Check sheet for the modelled part. Datum: model origin and axes. Units: mm. A direction names the side the tool comes from. Round coordinates to 2 decimals unless told otherwise and drop trailing zeros. Order: outer loops, then holes, each group sorted by start corner. A loop starts at its lowest first (then second) coordinate and runs counter-clockwise, first axis right, second up.
```python
from build123d import *

# Parameters (mm, degrees)
F2_R = 0.13


# Not quite as in the source:
# - a feature names something its author has since deleted; it is built from what else it names


with BuildPart() as f1:
    # F0 (on Top) → F1 (revolve)
    with BuildSketch(Plane.XY):
        with BuildLine():
            Line((7.3, 15.1), (7.3, 22.16))
            Line((7.3, 22.16), (1.6, 22.16))
            Line((1.6, 22.16), (1.6, 20.79))
            Line((1.6, 20.79), (2.9, 20.79))
            Line((2.9, 20.79), (2.9, 19.05))
            Line((2.9, 19.05), (3.16, 19.05))
            ThreePointArc((3.16, 19.05), (5.2813203436, 18.1713203436), (6.16, 16.05))
            Line((6.16, 16.05), (6.16, 15.1))
            Line((6.16, 15.1), (7.3, 15.1))
        make_face()
    revolve(axis=Axis((7.0380799007, 0, 0), (1, 0, 0)))

    # F2
    f2_edges = [f1.edges().sort_by_distance(p)[0] for p in [
        (7.3, -22.16, 0),
        (1.6, -22.16, 0),
        (1.6, -20.79, 0),
    ]]
    fillet(f2_edges, radius=F2_R)


solid = f1.part
```
Item 1: Sectioned sample at C-C (x = 5.55). Record the cut outline in (y, z), and give its area (3 significant figures).
Answer:
outline: circle Ø44.32 at (0, 0); hole circle Ø35.73 at (0, 0)
area: 540 mm2
Item 2: Release check for a two-part mould opening along Z. For faces 3 (the cylindrical face through (2.32, 19.83, 6.24)), 4 (the cylindrical face through (4.412, 21.137, 6.656)), 5 (the flat face through (1.6, 19.5, -8.1)) record: released by +Z, released by -Z, zero draft, split by the parting line, or undercut.
Answer:
face 3: undercut
face 4: split by the parting line
face 5: zero draft
Item 3: Access from +Z, -Z, +X, -X, +Y, -Y to the whole of each face (thin tool, end or side, straight path). Record for faces 1 (the cylindrical face through (6.74, -3.27, -14.74)), 2 (the flat face through (2.9, 9, -17)).
Answer:
face 1: +X, -X
face 2: -X
Item 4: Sectioned sample at A-A (z = 0). Record the cut outline in (x, y).
Answer:
outline: (1.6, -22.03) arc R0.13 ccw to (1.73, -22.16) - (7.17, -22.16) arc R0.13 ccw to (7.3, -22.03) - (7.3, -15.1) - (6.16, -15.1) - (6.16, -16.05) arc R3 cw to (3.16, -19.05) - (2.9, -19.05) - (2.9, -20.79) - (1.73, -20.79) arc R0.13 ccw to (1.6, -20.92) - close; (1.6, 20.92) arc R0.13 ccw to (1.73, 20.79) - (2.9, 20.79) - (2.9, 19.05) - (3.16, 19.05) arc R3 cw to (6.16, 16.05) - (6.16, 15.1) - (7.3, 15.1) - (7.3, 22.03) arc R0.13 ccw to (7.17, 22.16) - (1.73, 22.16) arc R0.13 ccw to (1.6, 22.03) - close
Item 5: Go/stop test with flat-tipped pins: P1, Ø3, axis at x = 3.5, z = -2.5, coming from the -Y side; P2, Ø2, axis at y = -14.5, z = 11, coming from the -X side. Record where each tip stops, or that it passes through.
Answer:
P1: stops at y = -22.14
P2: stops at x = 2.9
Item 6: Scan lines: line 1 along Z through (x, y) = (3.05, 0); line 2 along Z through (x, y) = (6.9, 0); line 3 along Y through (x, z) = (3.2, 2). Record each from-to range of solid material in increasing order.
Answer:
line 1: z = -22.16 to -19.05, 19.05 to 22.16
line 2: z = -22.16 to -15.1, 15.1 to 22.16
line 3: y = -22.07 to -18.94, 18.94 to 22.07
